Source: CAD feature listing. Evaluate the final solid. Frame: model axes, mm. Give positions to 0.01 mm unless a question says otherwise; leave off trailing zeros. Write item = value, one per line.
from build123d import *

# Parameters (mm, degrees)
BOSS_EXTRUDE1_DEPTH = 9
SKETCH2_R           = 1.09
CUT_EXTRUDE1_DEPTH  = 128.597021909
SKETCH3_R           = 1.5
CUT_EXTRUDE2_DEPTH  = 128.597021909


with BuildPart() as part:
    # Sketch1 → Boss-Extrude1 (new body)
    with BuildSketch(Plane(origin=(0, 0, 0), x_dir=(1, 0, 0), z_dir=(0, 1, 0))):
        with BuildLine():
            Line((-65, -90), (65, -90))
            ThreePointArc((65, -90), (82.67766953, -82.67766953), (90, -65))
            Line((90, -65), (90, 65))
            ThreePointArc((90, 65), (82.67766953, 82.67766953), (65, 90))
            Line((65, 90), (-65, 90))
            ThreePointArc((-65, 90), (-82.67766953, 82.67766953), (-90, 65))
            Line((-90, 65), (-90, -65))
            ThreePointArc((-90, -65), (-82.67766953, -82.67766953), (-65, -90))
        make_face()
    extrude(amount=BOSS_EXTRUDE1_DEPTH)

    # Sketch2 → Cut-Extrude1 (cut, through all)
    with BuildSketch(Plane(origin=(0, 9, 0), x_dir=(1, 0, 0), z_dir=(0, 1, 0))):
        with Locations(Location((-7.747, 70, 0), (0, 0, 270))):
            Circle(SKETCH2_R)
        with Locations(Location((7.747, 70, 0), (0, 0, 270))):
            Circle(SKETCH2_R)
    extrude(amount=-CUT_EXTRUDE1_DEPTH, mode=Mode.SUBTRACT)

    # Sketch3 → Cut-Extrude2 (cut, through all)
    with BuildSketch(Plane(origin=(0, 9, 0), x_dir=(1, 0, 0), z_dir=(0, 1, 0))):
        with Locations(Location((-65, 80, 0), (0, 0, 270))):
            Circle(SKETCH3_R)
        with Locations(Location((-80, 65, 0), (0, 0, 270))):
            Circle(SKETCH3_R)
        with Locations(Location((80, 65, 0), (0, 0, 270))):
            Circle(SKETCH3_R)
        with Locations(Location((80, -65, 0), (0, 0, 270))):
            Circle(SKETCH3_R)
        with Locations(Location((65, 80, 0), (0, 0, 270))):
            Circle(SKETCH3_R)
        with Locations(Location((65, -80, 0), (0, 0, 270))):
            Circle(SKETCH3_R)
        with Locations(Location((-65, -80, 0), (0, 0, 270))):
            Circle(SKETCH3_R)
        with Locations(Location((-80, -65, 0), (0, 0, 270))):
            Circle(SKETCH3_R)
    extrude(amount=-CUT_EXTRUDE2_DEPTH, mode=Mode.SUBTRACT)


solid = part.part
1. First-contact query: pin 1 Ø4 at (x, y) = (69, 8) entering from +Z. Flat tip, straight axial feed; report the tip coordinate or a pass-through.
Derived:
pin_1 = 89.92
2. Cut plane A-A, the plane y = 6.25. Count the separate pieces of the cut face and the enclosed holes in it, then the cut area to 3 significant figures.
Derived:
separate_pieces = 1
enclosed_holes = 10
area = 31,800 mm²
3. Material intervals for probe 1 along Z at (x, y) = (-65, 3.5); probe 2 along X at (y, z) = (4.75, 80), sorted ascending. Write a range as from..to.
Derived:
probe_1 = -90..-81.5, -78.5..78.5, 81.5..90
probe_2 = -85..-66.5, -63.5..63.5, 66.5..85
